from build123d import *

# Parameters (mm, degrees)
BOSS_EXTRUDE1_DEPTH = 9.525
CUT_EXTRUDE1_START  = -4.445
CUT_EXTRUDE1_DEPTH  = 4.445
SKETCH4_R           = 1.905
CUT_EXTRUDE2_DEPTH  = 228.118627562


with BuildPart() as part:
    # Sketch1 → Boss-Extrude1 (new body)
    with BuildSketch(Plane.XY):
        with BuildLine():
            Line((0, 0), (0, 25.4))
            Line((0, 25.4), (-22.86, 25.4))
            Line((-22.86, 25.4), (17.910019334, 215.579524422))
            Line((17.910019334, 215.579524422), (30.10047331, 222.402553944))
            ThreePointArc((30.10047331, 222.402553944), (36.413450877, 222.339405473), (39.551850365, 216.861438501))
            Line((39.551850365, 216.861438501), (41.637943134, 210.86387925))
            Line((41.637943134, 210.86387925), (6.35, 46.256543942))
            Line((6.35, 46.256543942), (6.35, 0))
            Line((6.35, 0), (0, 0))
        make_face()
    extrude(amount=BOSS_EXTRUDE1_DEPTH)

    # Sketch2 → Cut-Extrude1 (cut)
    with BuildSketch(Plane(origin=(0, 0, 0), x_dir=(-1, 0, 0), z_dir=(0, 0, -1)).offset(CUT_EXTRUDE1_START)):
        with BuildLine():
            Line((-41.637943134, 210.86387925), (-39.551850365, 216.861438501))
            ThreePointArc((-39.551850365, 216.861438501), (-31.336031581, 222.931135385), (-27.948316423, 213.29452371))
            Line((-27.948316423, 213.29452371), (-38.748816351, 197.386996815))
            Line((-38.748816351, 197.386996815), (-41.637943134, 210.86387925))
        make_face()
    extrude(amount=CUT_EXTRUDE1_DEPTH, mode=Mode.SUBTRACT)

    # Sketch4 → Cut-Extrude2 (cut, through all)
    with BuildSketch(Plane(origin=(0, 0, 4.445), x_dir=(-1, 0, 0), z_dir=(0, 0, -1))):
        with Locations((-36.399614201, 209.250963387)):
            Circle(SKETCH4_R)
        Polygon((-29.044835385, 218.558635146), (-31.50465372, 212.70442352), (-37.358865346, 215.164241855), (-34.89904701, 221.018453481), align=None)
    extrude(amount=-CUT_EXTRUDE2_DEPTH, mode=Mode.SUBTRACT)


solid = part.part
CAD build for the part. Positions are in the model's coordinates, mm. A direction names the side the tool comes from. Give positions to 0.01 mm unless a question says otherwise; leave off trailing zeros. Write each loop counter-clockwise with the first axis right and the second up, starting at its lowest first coordinate (ties: lowest second). Pieces come first, ordered by that corner, then holes. Notation, with made-up numbers: (89.25, -11.75) - (128.25, -11.75) arc R21 ccw to (128.25, 14.25) - close; hole circle Ø9 at (-10, -3). An arc over 180 degrees is marked (long way). Put each result on its own line as item: value.
(1) Pull direction Y, two halves, no side cores. Call faces 1 (the flat face through (3, 0, 5)), 2 (the flat face through (10, 120, 9.525)), 3 (the flat face through (34.391, 213.917, 6.949)): released by +Y, released by -Y, zero draft, split by the parting line, or undercut.
Working result:
face 1: released by -Y
face 2: zero draft
face 3: undercut
(2) Saw through at B-B (x = 2.5). List the corners of the cut face in (y, z) (3 decimals).
Working result:
outline: (0, 0) - (143.697, 0) - (143.697, 9.525) - (0, 9.525) - close
(3) Drop flat-ended pins along their axis: pin 1 Ø5 at (x, z) = (-7.5, 7) entering from -Y; pin 2 Ø4.5 at (x, y) = (37, 208) entering from -Z (3 decimals); pin 3 Ø2 at (x, y) = (26, 126.5) entering from -Z. Give the stop position or say it passes through.
Working result:
pin 1: y = 25.4
pin 2: z = 4.445
pin 3: through
(4) Wall check: L1, parallel to X at y = 213, z = 8; L2, parallel to X at y = 16, z = 2.5; L3, parallel to X at y = 42, z = 4. Give the ranges that are in metal, low to high.
Working result:
L1: 17.36 to 31.38, 32.21 to 40.89
L2: 0 to 6.35
L3: -19.3 to 6.35
(5) Saw through at C-C (y = 150). List the corners of the cut face in (x, z) (3 decimals).
Working result:
outline: (3.851, 0) - (28.59, 0) - (28.59, 9.525) - (3.851, 9.525) - close
(6) Tool access for faces 4 (the flat face through (6.35, 23, 5)), 5 (the flat face through (-11, 25.4, 5)), 6 (the flat face through (36.146, 218.05, 6.949)), 7 (the flat face through (36, 213, 4.445)): list every direction of +Z, -Z, +X, -X, +Y, -Y with a clear straight run to the whole face (end or side of a thin tool).
Working result:
face 4: +Z, -Z, +X, -Y
face 5: +Z, -Z, -X, -Y
face 6: +Z, -Z
face 7: -Z, +X
(7) Saw through at A-A (z = 6.25). List the corners of the cut face in (x, y) (3 decimals), then the cut area to 3 significant figures.
Working result:
outline: (-22.86, 25.4) - (0, 25.4) - (0, 0) - (6.35, 0) - (6.35, 46.257) - (41.638, 210.864) - (39.552, 216.861) arc R6.35 ccw to (30.1, 222.403) - (17.91, 215.58) - close; hole (29.045, 218.559) - (31.505, 212.704) - (37.359, 215.164) - (34.899, 221.018) - close; hole circle Ø3.81 at (36.4, 209.251)
area: 4,960 mm^2
